from build123d import *

# Parameters (mm, degrees)
F2_R           = 4.5
F2_W           = 20.8794145286
F2_H           = 3.3811966982
F3_DEPTH       = 6
F4_D           = 10
F4_DEPTH       = 4
F4_CBORE_D     = 12
F4_CBORE_DEPTH = 2
F4_TIP         = 3.0043030951
F6_D           = 9
F6_DEPTH       = 6
F6_CBORE_D     = 16
F6_CBORE_DEPTH = 2
F6_TIP         = 2.7038727856


with BuildPart() as f3:
    # F2 (on face) → F3 (new body)
    with BuildSketch(Plane.XZ):
        with BuildLine():
            Line((-74.1205854714, 17), (-93, 17))
            ThreePointArc((-93, 17), (-94.4142135624, 16.4142135624), (-95, 15))
            Line((-95, 15), (-95, 2.5))
            Line((-95, 2.5), (-74.1205854714, 2.5))
            Line((-74.1205854714, 2.5), (-74.1205854714, 17))
        make_face()
        with Locations((-83, 10)):
            Circle(F2_R, mode=Mode.SUBTRACT)
        Polygon((-95, 17), (-93, 17), (-74.1205854714, 17), (-74.1205854714, 22), (-95, 22), align=None)
        with Locations((-84.5602927357, 0.8094016509)):
            Rectangle(F2_W, F2_H)
        with Locations((-83, 10)):
            Circle(F2_R)
        with BuildLine():
            ThreePointArc((-95, 15), (-94.4142135624, 16.4142135624), (-93, 17))
            Line((-93, 17), (-95, 17))
            Line((-95, 17), (-95, 15))
        make_face()
    extrude(amount=F3_DEPTH)

    # F4
    with Locations(Plane(origin=(0, 0, 0), x_dir=(1, 0, 0), z_dir=(0, 1, 0))):
        with Locations((-63, -10), (-83, -10), (-83, 10), (-63, 10)):
            CounterBoreHole(F4_D / 2, F4_CBORE_D / 2, F4_CBORE_DEPTH, depth=F4_DEPTH)
            with Locations((0, 0, -(F4_DEPTH + F4_TIP / 2))):  # 118° drill point
                Cone(0, F4_D / 2, F4_TIP, mode=Mode.SUBTRACT)

    # F6
    with Locations(Plane.XZ.offset(6)):
        with Locations((-83, 10)):
            CounterBoreHole(F6_D / 2, F6_CBORE_D / 2, F6_CBORE_DEPTH, depth=F6_DEPTH)
            with Locations((0, 0, -(F6_DEPTH + F6_TIP / 2))):  # 118° drill point
                Cone(0, F6_D / 2, F6_TIP, mode=Mode.SUBTRACT)


solid = f3.part
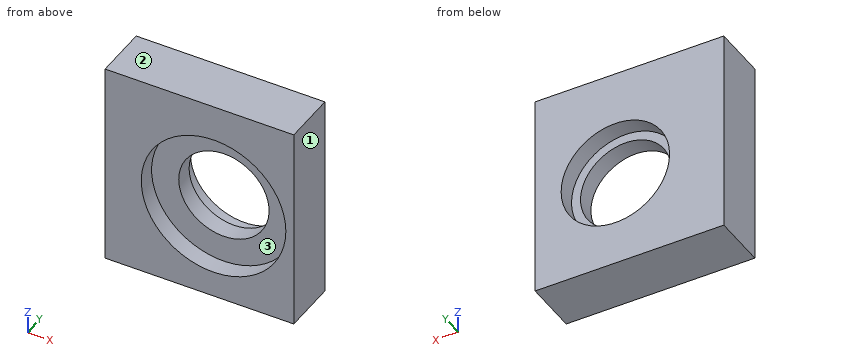
Here's how the part is built. I have some questions about the finished solid (model axes, mm). Face numbers are marked on the shaded views. Coordinates: 2 decimals unless noted, no trailing zeros. Order: outer loops, then holes, each group sorted by start corner. A loop starts at its lowest first (then second) coordinate and runs counter-clockwise, first axis right, second up.
Item 1: If we section it at C-C on z = 10: List the corners of the cut face in (x, y) for me.
Result sheet:
outline: (-95, -6) - (-91, -6) - (-91, -4) - (-88, -4) - (-88, -2) - (-89, -2) - (-89, 0) - (-95, 0) - close; (-78, -4) - (-75, -4) - (-75, -6) - (-74.12, -6) - (-74.12, 0) - (-77, 0) - (-77, -2) - (-78, -2) - close
Item 2: If we section it at B-B on y = -4.4: List the corners of the cut face in (x, z) for me, plus the area to 3 significant figures.
Result sheet:
outline: (-95, -0.88) - (-74.12, -0.88) - (-74.12, 22) - (-95, 22) - close; hole circle Ø16 at (-83, 10)
area: 277 mm2
Item 3: I need wall thicknesses on line 1 (Z direction, x = -83, y = -1.25); line 2 (Z direction, x = -83, y = -3.6); line 3 (Y direction, x = -78, z = 15.25). Which ranges of each line are inside material? Lowest first, please.
Result sheet:
line 1: z = -0.88 to 4, 16 to 22
line 2: z = -0.88 to 5, 15 to 22
line 3: y = -4 to 0
Item 4: If we section it at D-D on x = -89.75: List the corners of the cut face in (y, z) for me, plus the area to 3 significant figures.
Result sheet:
outline: (-6, -0.88) - (0, -0.88) - (0, 22) - (-6, 22) - (-6, 14.29) - (-4, 14.29) - (-4, 5.71) - (-6, 5.71) - close
area: 120 mm2
Item 5: If we section it at A-A on x = -83: List the corners of the cut face in (y, z) for me, plus the area to 3 significant figures.
Result sheet:
outline: (-6, -0.88) - (0, -0.88) - (0, 4) - (-2, 4) - (-2, 5) - (-4, 5) - (-4, 2) - (-6, 2) - close; (-6, 18) - (-4, 18) - (-4, 15) - (-2, 15) - (-2, 16) - (0, 16) - (0, 22) - (-6, 22) - close
area: 61.3 mm2
Item 6: If we mould it in two halves opening along X, with no side actions, what happens to the marked faces 1, 2 and 3? For each: +X half, -X half, draft (parallel to the pull), parting line (faces both ways), or undercut.
Result sheet:
face 1: +X half
face 2: draft
face 3: undercut
